from build123d import *

# Parameters (mm, degrees)
F1_DEPTH  = 3.048
F2_R      = 30.5
F2_R_2    = 46.5
F2_R_3    = 1.524
F3_DEPTH  = 25.4
F4_W      = 115.7319251503
F4_H      = 3.048
F5_DEPTH  = 3.049
F7_W      = 2.54
F7_H      = 0.254
F8_DEPTH  = 3.049
F10_DEPTH = 3.048
F11_W     = 3.175
F11_H     = 1.524
F12_DEPTH = 1.5875


with BuildPart() as f1:
    # F0 (on Top) → F1 (new body)
    with BuildSketch(Plane.XY):
        with BuildLine():
            Line((-79.9225977639, 113.03), (-137.8481502717, 12.7))
            ThreePointArc((-137.8481502717, 12.7), (-141.2511050156, 0), (-137.8481502717, -12.7))
            Line((-137.8481502717, -12.7), (-79.9225977639, -113.03))
            ThreePointArc((-79.9225977639, -113.03), (-70.6255525078, -122.3270452561), (-57.9255525078, -125.73))
            Line((-57.9255525078, -125.73), (57.9255525078, -125.73))
            ThreePointArc((57.9255525078, -125.73), (70.6255525078, -122.3270452561), (79.9225977639, -113.03))
            Line((79.9225977639, -113.03), (137.8481502717, -12.7))
            ThreePointArc((137.8481502717, -12.7), (141.2511050156, 0), (137.8481502717, 12.7))
            Line((137.8481502717, 12.7), (79.9225977639, 113.03))
            ThreePointArc((79.9225977639, 113.03), (70.6255525078, 122.3270452561), (57.9255525078, 125.73))
            Line((57.9255525078, 125.73), (-57.9255525078, 125.73))
            ThreePointArc((-57.9255525078, 125.73), (-70.6255525078, 122.3270452561), (-79.9225977639, 113.03))
        make_face()
    extrude(amount=F1_DEPTH)

    # F2 (on face) → F3 (cut)
    with BuildSketch(Plane.XY.offset(3.048)):
        with Locations((0, 62.23)):
            Circle(F2_R)
        with Locations((0, -49.53)):
            Circle(F2_R_2)
        with Locations((57.15, -49.53)):
            Circle(F2_R_3)
        with Locations((30.2848859509, -1.0640513047)):
            Circle(F2_R_3)
        with Locations((30.2848859509, -97.9959486953)):
            Circle(F2_R_3)
        with Locations((-30.2848859509, -1.0640513047)):
            Circle(F2_R_3)
        with Locations((-30.2848859509, -97.9959486953)):
            Circle(F2_R_3)
        with Locations((-57.15, -49.53)):
            Circle(F2_R_3)
        with Locations((-27.559, 89.789)):
            Circle(F2_R_3)
        with Locations((-27.559, 34.671)):
            Circle(F2_R_3)
        with Locations((27.559, 34.671)):
            Circle(F2_R_3)
        with Locations((27.559, 89.789)):
            Circle(F2_R_3)
    extrude(amount=-F3_DEPTH, mode=Mode.SUBTRACT)

    # F4 (on face) → F5 (cut, through all)
    with BuildSketch(Plane.XY.offset(3.048)):
        Polygon((-135.0389296821, -11.215712791), (-77.1729671069, -111.4425), (-74.5333216761, -109.9185), (-132.3992842513, -9.6917127909), align=None)
        Polygon((-77.2325570395, 111.339287209), (-135.0985196147, 11.1125), (-132.4588741839, 9.5885), (-74.5929116088, 109.8152872091), align=None)
        with Locations((-0.0595899326, 121.031)):
            Rectangle(F4_W, F4_H)
        Polygon((135.0389296821, 11.215712791), (77.1729671069, 111.4425), (74.5333216761, 109.9185), (132.3992842513, 9.691712791), align=None)
        Polygon((77.2325570395, -111.339287209), (135.0985196147, -11.1125), (132.4588741839, -9.5885), (74.5929116088, -109.815287209), align=None)
        with Locations((0.0595899326, -121.031)):
            Rectangle(F4_W, F4_H)
    extrude(amount=-F5_DEPTH, mode=Mode.SUBTRACT)

    # F7 (on face) → F8 (cut, through all)
    with BuildSketch(Plane.XY.offset(3.048)):
        with Locations((-9.525, -125.603)):
            Rectangle(F7_W, F7_H)
        with Locations((9.5845899326, -125.603)):
            Rectangle(F7_W, F7_H)
    extrude(amount=-F8_DEPTH, mode=Mode.SUBTRACT)

    # F9 (on face) → F10 (join)
    with BuildSketch(Plane.XY.offset(3.048)):
        with BuildLine():
            Line((-73.3234841871, 124.46), (-79.9225977639, 113.03))
            Line((-79.9225977639, 113.03), (-57.9255525078, 125.73))
            Line((-57.9255525078, 125.73), (-71.1237796615, 125.73))
            ThreePointArc((-71.1237796615, 125.73), (-72.3937796615, 125.3897045256), (-73.3234841871, 124.46))
        make_face()
        with BuildLine():
            ThreePointArc((-137.8481502717, -12.7), (-141.2511050156, 0), (-137.8481502717, 12.7))
            Line((-137.8481502717, 12.7), (-144.4472638486, 1.27))
            ThreePointArc((-144.4472638486, 1.27), (-144.7875593229, 0), (-144.4472638486, -1.27))
            Line((-144.4472638486, -1.27), (-137.8481502717, -12.7))
        make_face()
        with BuildLine():
            ThreePointArc((-57.9255525078, -125.73), (-70.6255525078, -122.3270452561), (-79.9225977639, -113.03))
            Line((-79.9225977639, -113.03), (-73.3234841871, -124.46))
            ThreePointArc((-73.3234841871, -124.46), (-72.3937796615, -125.3897045256), (-71.1237796615, -125.73))
            Line((-71.1237796615, -125.73), (-57.9255525078, -125.73))
        make_face()
        with BuildLine():
            Line((73.3234841871, -124.46), (79.9225977639, -113.03))
            ThreePointArc((79.9225977639, -113.03), (70.6255525078, -122.3270452561), (57.9255525078, -125.73))
            Line((57.9255525078, -125.73), (71.1237796615, -125.73))
            ThreePointArc((71.1237796615, -125.73), (72.3937796615, -125.3897045256), (73.3234841871, -124.46))
        make_face()
        with BuildLine():
            Line((144.4472638486, 1.27), (137.8481502717, 12.7))
            ThreePointArc((137.8481502717, 12.7), (141.2511050156, 0), (137.8481502717, -12.7))
            Line((137.8481502717, -12.7), (144.4472638486, -1.27))
            ThreePointArc((144.4472638486, -1.27), (144.7875593229, 0), (144.4472638486, 1.27))
        make_face()
        with BuildLine():
            Line((71.1237796615, 125.73), (57.9255525078, 125.73))
            ThreePointArc((57.9255525078, 125.73), (70.6255525078, 122.3270452561), (79.9225977639, 113.03))
            Line((79.9225977639, 113.03), (73.3234841871, 124.46))
            ThreePointArc((73.3234841871, 124.46), (72.3937796615, 125.3897045256), (71.1237796615, 125.73))
        make_face()
    extrude(amount=-F10_DEPTH)

    # F11 (on face) → F12 (cut)
    with BuildSketch(Plane.XY.offset(3.048)):
        with BuildLine():
            Line((-57.9255525078, 117.983), (-57.9255525078, 119.507))
            ThreePointArc((-57.9255525078, 119.507), (-67.5657049473, 116.9079552121), (-74.5929116088, 109.8152872091))
            Line((-74.5929116088, 109.8152872091), (-73.2684038811, 109.0614601206))
            ThreePointArc((-73.2684038811, 109.0614601206), (-66.7996293906, 115.5904939256), (-57.9255525078, 117.983))
        make_face()
        with Locations((-56.3380525078, 118.745)):
            Rectangle(F11_W, F11_H)
        Polygon((-73.2684038811, 109.0614601206), (-74.5929116088, 109.8152872091), (-76.1804116088, 107.065656552), (-74.8388469782, 106.3021217395), align=None)
        with BuildLine():
            Line((73.2182344036, 109.1483562046), (74.5333216761, 109.9185))
            ThreePointArc((74.5333216761, 109.9185), (67.446525082, 116.9398894425), (57.8063726425, 119.507))
            Line((57.8063726425, 119.507), (57.8063726425, 117.983))
            ThreePointArc((57.8063726425, 117.983), (66.6886079177, 115.6177179059), (73.2182344036, 109.1483562046))
        make_face()
        Polygon((76.1208216761, 107.168869343), (74.5333216761, 109.9185), (73.2182344036, 109.1483562046), (74.801024176, 106.406883901), align=None)
        with Locations((56.2188726425, 118.745)):
            Rectangle(F11_W, F11_H)
        with BuildLine():
            Line((-131.1390514686, 8.8265), (-132.4588741839, 9.5885))
            ThreePointArc((-132.4588741839, 9.5885), (-135.0281115918, -0.0596393029), (-132.3992842513, -9.6917127909))
            Line((-132.3992842513, -9.6917127909), (-131.0841969788, -8.9215689955))
            ThreePointArc((-131.0841969788, -8.9215689955), (-133.5041188708, -0.0549290528), (-131.1390514686, 8.8265))
        make_face()
        Polygon((-130.8713741839, 12.338130657), (-132.4588741839, 9.5885), (-131.1390514686, 8.8265), (-129.563948664, 11.5940256944), align=None)
        Polygon((-131.0841969788, -8.9215689955), (-132.3992842513, -9.6917127909), (-130.8117842513, -12.4413434479), (-129.4919867512, -11.679358006), align=None)
        with BuildLine():
            Line((-73.2134989608, -109.1565), (-74.5333216761, -109.9185))
            ThreePointArc((-74.5333216761, -109.9185), (-67.4624066445, -116.9675945149), (-57.8063726425, -119.507))
            Line((-57.8063726425, -119.507), (-57.8157930976, -117.983029116))
            ThreePointArc((-57.8157930976, -117.983029116), (-66.7044894803, -115.6454229784), (-73.2134989608, -109.1565))
        make_face()
        Polygon((-76.1208216761, -107.1688693429), (-74.5333216761, -109.9185), (-73.2134989608, -109.1565), (-74.8009989608, -106.4068693429), align=None)
        Polygon((-57.8157930976, -117.983029116), (-57.8063726425, -119.507), (-54.6313726425, -119.507), (-54.6313726425, -117.983029116), align=None)
        with BuildLine():
            Line((57.9161320527, -117.983029116), (57.9255525078, -119.507))
            ThreePointArc((57.9255525078, -119.507), (67.5496524319, -116.8803488392), (74.5929116088, -109.815287209))
            Line((74.5929116088, -109.815287209), (73.2730888934, -109.053287209))
            ThreePointArc((73.2730888934, -109.053287209), (66.7835768752, -115.5628875527), (57.9161320527, -117.983029116))
        make_face()
        Polygon((54.7505525078, -119.507), (57.9255525078, -119.507), (57.9161320527, -117.983029116), (54.7505525078, -117.983029116), align=None)
        Polygon((73.2730888934, -109.053287209), (74.5929116088, -109.815287209), (76.1804116088, -107.065656552), (74.8605888934, -106.303656552), align=None)
        with BuildLine():
            Line((131.1343664563, -8.8346729115), (132.4588741839, -9.5885))
            ThreePointArc((132.4588741839, -9.5885), (134.9961775139, 0.0595406033), (132.3992842513, 9.691712791))
            Line((132.3992842513, 9.691712791), (131.0794615359, 8.929712791))
            ThreePointArc((131.0794615359, 8.929712791), (133.4721847929, 0.0548303532), (131.1343664563, -8.8346729115))
        make_face()
        Polygon((130.8713741839, -12.338130657), (132.4588741839, -9.5885), (131.1343664563, -8.8346729115), (129.5515766838, -11.576145215), align=None)
        Polygon((131.0794615359, 8.929712791), (132.3992842513, 9.691712791), (130.8117842513, 12.441343448), (129.4919615359, 11.679343448), align=None)
    extrude(amount=-F12_DEPTH, mode=Mode.SUBTRACT)


solid = f1.part
Verification items for the finished model (mm, model axes). A direction names the side the tool comes from. Coordinates: 2 decimals unless noted, no trailing zeros. Write each loop counter-clockwise with the first axis right and the second up, starting at its lowest first coordinate (ties: lowest second). Pieces come first, ordered by that corner, then holes. Notation, with made-up numbers: (28.25, -24.5) - (81.25, -24.5) arc R20 ccw to (81.25, -8.5) - close; hole circle Ø5 at (-15.75, 36). An arc over 180 degrees is marked (long way). Answer as a JSON object with one key per item and string values.
(1) Cross-section at D-D on z = 0.5. Give the number of separate pieces and of enclosed holes in the cut face, plus the area to 3 significant figures.
Report:
{"separate pieces": "1", "enclosed holes": "18", "area": "42,900 mm^2"}
(2) Tool access check on faces 3 (the flat face through (105.76, -61.93, 1.55)), 4 (the flat face through (-2, 2, 3.048)), 5 (the cylindrical face through (66.896, -115.497, 2.265)). Record the directions out of +Z, -Z, +X, -X, +Y, -Y that give a thin tool (end or side, any length) a straight path to the whole face; none if there is none.
Report:
{"face 3": "+Z, -Z", "face 4": "+Z, +X, -X, +Y, -Y", "face 5": "+Z"}
(3) Cross-section at A-A on x = 0. Record the cut outline in (y, z) (3 decimals), plus the area to 3 significant figures.
Report:
{"outline": "(-125.73, 0) - (-122.555, 0) - (-122.555, 3.048) - (-125.73, 3.048) - close; (-119.507, 0) - (-96.03, 0) - (-96.03, 3.048) - (-119.507, 3.048) - close; (-3.03, 0) - (31.73, 0) - (31.73, 3.048) - (-3.03, 3.048) - close; (92.73, 0) - (119.507, 0) - (119.507, 3.048) - (92.73, 3.048) - close; (122.555, 0) - (125.73, 0) - (125.73, 3.048) - (122.555, 3.048) - close", "area": "278 mm^2"}
(4) Gauge pin test, flat ends, axial feed: pin 1 Ø4 at (x, y) = (-30.28, -98) entering from +Z; pin 2 Ø1.2 at (y, z) = (-118.5, 2.5) entering from -X; pin 3 Ø0.5 at (y, z) = (119, 2) entering from -X. Record the tip position at first contact, or that the pin passes through.
Report:
{"pin 1": "z = 3.05", "pin 2": "x = -77.11", "pin 3": "x = -76.62"}
(5) Thickness scan on line 1 along Y through (x, z) = (-52.5, 1.85) (3 decimals); line 2 along X through (y, z) = (53, 1.5); line 3 along X through (y, z) = (40, 2.15). Record the ranges inside material, lowest first.
Report:
{"line 1": "-125.73 to -122.555, -119.507 to 119.507, 122.555 to 125.73", "line 2": "-114.58 to -110.91, -107.4 to -29.07, 29.07 to 107.4, 110.91 to 114.58", "line 3": "-122.09 to -118.42, -114.9 to -20.88, 20.88 to 114.9, 118.42 to 122.09"}
(6) Cross-section at B-B on x = -96. Record the cut outline in (y, z), plus the area to 3 significant figures.
Report:
{"outline": "(-85.18, 0) - (-78.83, 0) - (-78.83, 3.05) - (-85.18, 3.05) - close; (-72.74, 0) - (72.74, 0) - (72.74, 3.05) - (-72.74, 3.05) - close; (78.83, 0) - (85.18, 0) - (85.18, 3.05) - (78.83, 3.05) - close", "area": "482 mm^2"}
(7) Mould release check, pull along Y, two halves, no side actions. Record for faces 1 (the flat face through (-2, 2, 0)), 2 (the cylindrical face through (67.43, -116.95, 2.27)): pulls with the +Y half, pulls with the -Y half, needs draft (parallel to the pull), parting line crosses it, or undercut.
Report:
{"face 1": "needs draft", "face 2": "undercut"}
(8) Cross-section at C-C on y = 40.5. Record the cut outline in (x, z).
Report:
{"outline": "(-121.8, 0) - (-118.13, 0) - (-118.13, 3.05) - (-121.8, 3.05) - close; (-114.61, 0) - (-21.4, 0) - (-21.4, 3.05) - (-114.61, 3.05) - close; (21.4, 0) - (114.61, 0) - (114.61, 3.05) - (21.4, 3.05) - close; (118.13, 0) - (121.8, 0) - (121.8, 3.05) - (118.13, 3.05) - close"}
